Model file for the job. Use its own axes, mm. Face numbers are marked on the shaded views. A direction names the side the tool comes from. Coordinates: 2 decimals unless noted, no trailing zeros. Write each loop counter-clockwise with the first axis right and the second up, starting at its lowest first coordinate (ties: lowest second). Pieces come first, ordered by that corner, then holes. Notation, with made-up numbers: M 52.5,-28 L 95.5,-28 A17 ccw 95.5,-17 Z; hole C 89.25,-37 d7. An arc over 180 degrees is marked long. One line per question, with ' | ' between items. Start each with the question number.
(1) Flat gauge pins, fed straight in: pin 1 Ø3 at (x, z) = (64, -1) entering from -Y; pin 2 Ø5 at (x, z) = (64.5, 0) entering from +Y; pin 3 Ø10 at (x, z) = (-34, 23.5) entering from +Y; pin 4 Ø8 at (x, z) = (-34.5, -14) entering from -Y. Where does each tip first touch, or does it go through?
(2) Cut at B-B (x = 32). Write the cut outline in (y, z), plus the area to 3 significant figures.
(3) Tool access for the marked faces 5, 6 and 7: list every direction of +Z, -Z, +X, -X, +Y, -Y with a clear straight run to the whole face (end or side of a thin tool).
(4) Two-plate mould, pull along Z, no slides. Class the marked faces 1, 2, 3 and 4: +Z half, -Z half, draft (parallel to the pull), parting line (faces both ways), or undercut.
(5) Cut at C-C (z = 19). Write the cut outline in (x, y), plus the area to 3 significant figures.
(6) Cut at A-A (y = 11.5). Write the cut outline in (x, z).
(7) Wall check: probe 1 along Z at (x, y) = (51.5, 11); probe 2 along X at (y, z) = (30.5, 32); probe 3 along X at (y, z) = (4.5, -29.5). Give the ranges that are in metal, low to high.
from build123d import *

# Parameters (mm, degrees)
SKETCH_1_W      = 120
SKETCH_1_H      = 70
EXTRUDE_1_DEPTH = 3
SKETCH_3_W      = 120
SKETCH_3_H      = 70
EXTRUDE_2_DEPTH = 33
EXTRUDE_3_DEPTH = 10


with BuildPart() as part:
    # 草图1 → 凸台-拉伸1 (new body)
    with BuildSketch(Plane(origin=(0, 0, 0), x_dir=(1, 0, 0), z_dir=(0, 1, 0))):
        Rectangle(SKETCH_1_W, SKETCH_1_H)
    extrude(amount=EXTRUDE_1_DEPTH)

    # 草图3 → 凸台-拉伸2 (add)
    with BuildSketch(Plane(origin=(0, 0, 0), x_dir=(1, 0, 0), z_dir=(0, 1, 0))):
        Rectangle(SKETCH_3_W, SKETCH_3_H)
        Polygon((-56.372128616, 32.883741693), (56.372128616, 32.883741693), (56.372128616, -32.883741693), (-55.8, -32.55), align=None, mode=Mode.SUBTRACT)
    extrude(amount=EXTRUDE_2_DEPTH)

    # 草图4 → 凸台-拉伸3 (add)
    with BuildSketch(Plane(origin=(60, 0, 0), x_dir=(0, 0, -1), z_dir=(1, 0, 0))):
        with BuildLine():
            Line((-5.198866843, 19.159885362), (5.03766167, 19.159885362))
            ThreePointArc((5.03766167, 19.159885362), (7.697547031, 16.5), (5.03766167, 13.840114638))
            Line((5.03766167, 13.840114638), (-5.198866843, 13.840114638))
            ThreePointArc((-5.198866843, 13.840114638), (-7.858752205, 16.5), (-5.198866843, 19.159885362))
        make_face()
    extrude(amount=EXTRUDE_3_DEPTH)


solid = part.part
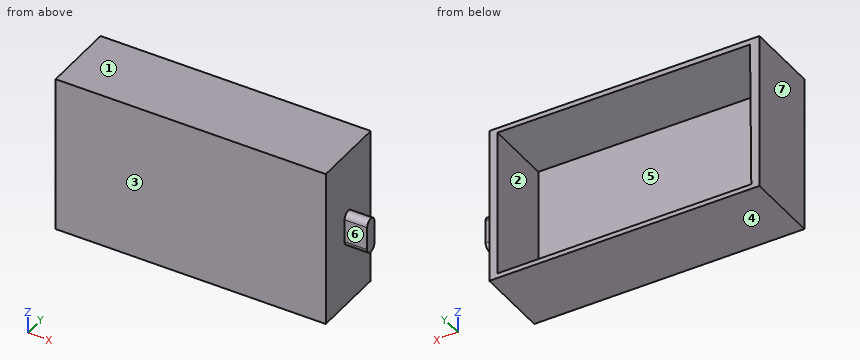
Filled in:
1) pin 1: y = 13.84 | pin 2: y = 19.16 | pin 3: y = 3 | pin 4: y = 0
2) outline: M 0,-35 L 33,-35 L 33,-32.88 L 3,-32.88 L 3,32.81 L 33,32.81 L 33,35 L 0,35 Z | area: 339 mm²
3) face 5: +Y | face 6: +Z, -Z, +X, -Y | face 7: +Z, -Z, -X, +Y, -Y
4) face 1: +Z half | face 2: undercut | face 3: draft | face 4: -Z half
5) outline: M -60,0 L 60,0 L 60,33 L 56.37,33 L 56.37,3 L -55.92,3 L -55.92,33 L -60,33 Z | area: 591 mm²
6) outline: M -60,-35 L 60,-35 L 60,35 L -60,35 Z; hole M -56.37,-32.88 L 56.37,-32.88 L 56.37,32.88 L -55.8,32.55 Z
7) probe 1: -35 to -32.88, 32.87 to 35 | probe 2: -60 to -55.8, 56.37 to 60 | probe 3: -60 to -56.34, 56.37 to 60
